Geometry: see drawing. Coordinates: mm, zero at the bounding-box minimum. A direction names the side the tool comes from. Coordinates: 2 decimals unless noted, no trailing zeros. Loops run counter-clockwise (first coordinate to the right, second up) from the corner with the lowest first, then second, coordinate; pieces in that order, holes last. Notation, with made-up numbers: M 0.25,-4 L 50.25,-4 A12 cw 50.25,4 Z; hole C -32,-32 d5. An arc over 180 degrees is marked long. One line per question, with ' | ' between items. Start each with the question number.
1. Section query A-A, the plane y = 25. Output: boundary loops of the cut face in (x, z).
2. Pin query (flat end, axial travel): P1, Ø8, axis at x = 16, y = 15.5, coming from the -Z side; P2, Ø2.5, axis at x = 5, z = 5, coming from the -Y side; P3, Ø4, axis at x = 13.25, y = 38.42, coming from the +Z side. Return the tip coordinate at first contact, or that it passes through.
3. Section query B-B, the plane x = 21. Output: boundary loops of the cut face in (y, z), and give its area (3 significant figures).
4. Ray query, probe 1 along Z at (x, y) = (37, 1.4); probe 2 along X at (y, z) = (1.1, 25); probe 3 along Y at (x, z) = (24, 34). Return the intervals inside material, ascending.
5. Access query for the marked faces 1 and 2. Directions: +Z, -Z, +X, -X, +Y, -Y. A direction counts if a zero-diameter tool reaches every point of the face in a straight line with its end or side. Return the directions, or none.
6. Section query C-C, the plane z = 45. Output: boundary loops of the cut face in (x, y).
7. Section query D-D, the plane x = 28.75. Output: boundary loops of the cut face in (y, z).
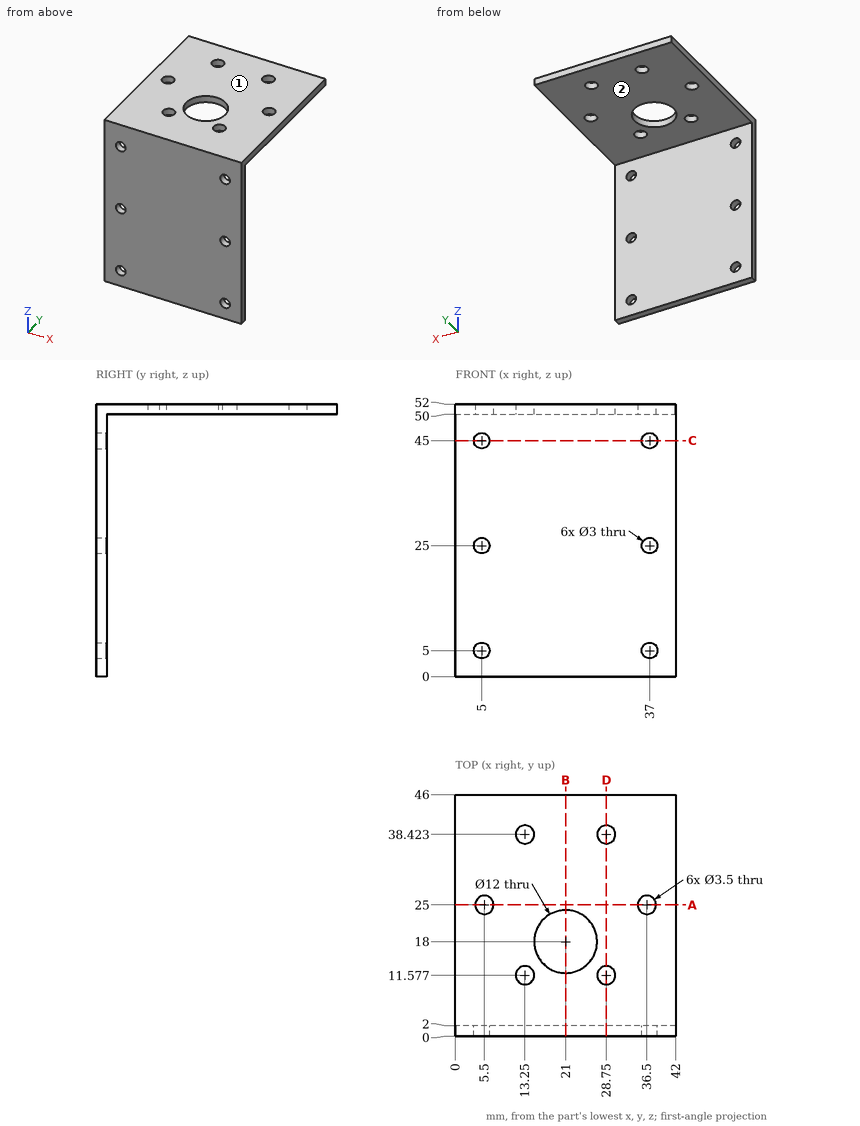
Taken from the geometry:
1) outline: M 0,50 L 3.75,50 L 3.75,52 L 0,52 Z; M 7.25,50 L 34.75,50 L 34.75,52 L 7.25,52 Z; M 38.25,50 L 42,50 L 42,52 L 38.25,52 Z
2) P1: z = 50 | P2: through | P3: z = 52
3) outline: M 0,0 L 2,0 L 2,50 L 12,50 L 12,52 L 0,52 Z; M 24,50 L 46,50 L 46,52 L 24,52 Z | area: 168 mm^2
4) probe 1: 0 to 3.5, 6.5 to 23.5, 26.5 to 43.5, 46.5 to 52 | probe 2: 0 to 3.5, 6.5 to 35.5, 38.5 to 42 | probe 3: 0 to 2
5) face 1: +Z, +X, -X, +Y, -Y | face 2: -Z, +X, -X, +Y
6) outline: M 0,0 L 3.5,0 L 3.5,2 L 0,2 Z; M 6.5,0 L 35.5,0 L 35.5,2 L 6.5,2 Z; M 38.5,0 L 42,0 L 42,2 L 38.5,2 Z
7) outline: M 0,0 L 2,0 L 2,50 L 9.83,50 L 9.83,52 L 0,52 Z; M 13.33,50 L 36.67,50 L 36.67,52 L 13.33,52 Z; M 40.17,50 L 46,50 L 46,52 L 40.17,52 Z
